The listing builds one solid part. Answer for the finished solid, in the listing's coordinates (mm). A direction names the side the tool comes from. Coordinates: 2 decimals unless noted, no trailing zeros. Write each loop counter-clockwise with the first axis right and the second up, starting at its lowest first coordinate (ties: lowest second). Pieces come first, ordered by that corner, then holes. Notation, with made-up numbers: M 19.25,62.25 L 71.25,62.25 A16 ccw 71.25,83.25 Z; hole C 23.25,-4 d6. An arc over 180 degrees is marked long. Write item = value, one per line. Start each with the question number.
```python
from build123d import *

# Parameters (mm, degrees)
EXTRUDE_1_DEPTH     = 3
SKETCH_3_W          = 60
SKETCH_3_H          = 31.5
EXTRUDE_2_DEPTH     = 2
SKETCH_4_R          = 0.5
CUT_EXTRUDE_1_DEPTH = 10
SKETCH_5_R          = 1.5
CUT_EXTRUDE_2_DEPTH = 10
SKETCH_6_W          = 5
SKETCH_6_H          = 31.5
EXTRUDE_3_DEPTH     = 48.15
EXTRUDE_START       = 5
SKETCH_7_R          = 1.6
EXTRUDE_4_DEPTH     = 5
CUT_EXTRUDE_3_DEPTH = 2
FILLET_1_R          = 2
FILLET_2_R          = 2
CUT_EXTRUDE_5_DEPTH = 1.6
SKETCH_11_R         = 0.5
SKETCH_11_R_2       = 1.5
EXTRUDE_5_DEPTH     = 3
SKETCH_12_W         = 31.5
SKETCH_12_H         = 1.6
EXTRUDE_6_DEPTH     = 9
FILLET_4_R          = 1.6
EXTRUDE_START_2     = 1.6
SKETCH_13_R         = 10
SKETCH_13_R_2       = 1.75
SKETCH_13_R_3       = 0.5
EXTRUDE_7_DEPTH     = 1.6
SKETCH_14_R         = 1.6
CUT_EXTRUDE_6_DEPTH = 67.6


with BuildPart() as part:
    # 草图1 → 凸台-拉伸1 (new body)
    with BuildSketch(Plane(origin=(0, 0, 0), x_dir=(1, 0, 0), z_dir=(0, 1, 0))):
        with BuildLine():
            Line((0, -15.75), (90, -15.75))
            Line((90, -15.75), (90, 15.75))
            Line((90, 15.75), (0, 15.75))
            ThreePointArc((0, 15.75), (-15.75, 0), (0, -15.75))
        make_face()
    extrude(amount=EXTRUDE_1_DEPTH)

    # 草图3 → 凸台-拉伸2 (add)
    with BuildSketch(Plane.XZ):
        with Locations((60, 0)):
            Rectangle(SKETCH_3_W, SKETCH_3_H)
    extrude(amount=EXTRUDE_2_DEPTH)

    # 草图4 → 切除-拉伸1 (cut)
    with BuildSketch(Plane.XZ):
        with Locations(Location((0, 7, 0), (0, 0, 270))):
            Circle(SKETCH_4_R)
        with Locations(Location((7, 0, 0), (0, 0, 270))):
            Circle(SKETCH_4_R)
        with Locations(Location((0, -7, 0), (0, 0, 270))):
            Circle(SKETCH_4_R)
        with Locations(Location((-7, 0, 0), (0, 0, 270))):
            Circle(SKETCH_4_R)
    extrude(amount=-CUT_EXTRUDE_1_DEPTH, mode=Mode.SUBTRACT)

    # 草图5 → 切除-拉伸2 (cut)
    with BuildSketch(Plane(origin=(0, 3, 0), x_dir=(1, 0, 0), z_dir=(0, 1, 0))):
        with Locations(Location((0, 0, 0), (0, 0, 270))):
            Circle(SKETCH_5_R)
    extrude(amount=-CUT_EXTRUDE_2_DEPTH, mode=Mode.SUBTRACT)

    # 草图6 → 凸台-拉伸3 (add)
    with BuildSketch(Plane.XZ.offset(2)):
        with Locations((87.5, 0)):
            Rectangle(SKETCH_6_W, SKETCH_6_H)
    extrude(amount=EXTRUDE_3_DEPTH)

    # 草图7 → 凸台-拉伸4 (add)
    with BuildSketch(Plane.XZ.offset(50.15).offset(EXTRUDE_START)):
        with BuildLine():
            Line((90, 15.75), (0, 15.75))
            ThreePointArc((0, 15.75), (-15.75, 0), (0, -15.75))
            Line((0, -15.75), (90, -15.75))
            Line((90, -15.75), (90, 15.75))
        make_face()
        with Locations(Location((8.03393099, 0, 0), (0, 0, 270))):
            Circle(SKETCH_7_R, mode=Mode.SUBTRACT)
        with Locations(Location((0, 8, 0), (0, 0, 270))):
            Circle(SKETCH_7_R, mode=Mode.SUBTRACT)
        with Locations(Location((0.03393099, -7.999928043, 0), (0, 0, 270))):
            Circle(SKETCH_7_R, mode=Mode.SUBTRACT)
        with Locations(Location((-8, 0, 0), (0, 0, 270))):
            Circle(SKETCH_7_R, mode=Mode.SUBTRACT)
    extrude(amount=-EXTRUDE_4_DEPTH)

    # 草图8 → 切除-拉伸3 (cut)
    with BuildSketch(Plane(origin=(0, -50.15, 0), x_dir=(1, 0, 0), z_dir=(0, 1, 0))):
        Polygon((0, 15.75), (30, 15.75), (30, -15.75), (0, -15.75), (-20, -15.75), (-20, 15.75), align=None)
    extrude(amount=-CUT_EXTRUDE_3_DEPTH, mode=Mode.SUBTRACT)

    # 圆角1
    fillet_1_edges = [part.edges().sort_by_distance(p)[0] for p in [
        (85, -2, 0),
    ]]
    fillet(fillet_1_edges, radius=FILLET_1_R)

    # 圆角2
    fillet_2_edges = [part.edges().sort_by_distance(p)[0] for p in [
        (85, -50.15, 0),
    ]]
    fillet(fillet_2_edges, radius=FILLET_2_R)

    # 草图10 → 切除-拉伸5 (cut)
    with BuildSketch(Plane.XZ):
        with BuildLine():
            Line((30, -15.75), (30, 15.75))
            Line((30, 15.75), (0, 15.75))
            ThreePointArc((0, 15.75), (-15.75, 0), (0, -15.75))
            Line((0, -15.75), (30, -15.75))
        make_face()
    extrude(amount=-CUT_EXTRUDE_5_DEPTH, mode=Mode.SUBTRACT)

    # 草图11 → 凸台-拉伸5 (add)
    with BuildSketch(Plane.XZ.offset(-1.6)):
        with BuildLine():
            Line((0, -15.75), (30, -15.75))
            Line((30, -15.75), (30, 15.75))
            Line((30, 15.75), (0, 15.75))
            ThreePointArc((0, 15.75), (-15.75, 0), (0, -15.75))
        make_face()
        with Locations(Location((0, -7, 0), (0, 0, 270))):
            Circle(SKETCH_11_R, mode=Mode.SUBTRACT)
        with Locations(Location((-7, 0, 0), (0, 0, 270))):
            Circle(SKETCH_11_R, mode=Mode.SUBTRACT)
        with Locations(Location((0, 0, 0), (0, 0, 270))):
            Circle(SKETCH_11_R_2, mode=Mode.SUBTRACT)
        with Locations(Location((0, 7, 0), (0, 0, 270))):
            Circle(SKETCH_11_R, mode=Mode.SUBTRACT)
        with Locations(Location((7, 0, 0), (0, 0, 270))):
            Circle(SKETCH_11_R, mode=Mode.SUBTRACT)
    extrude(amount=-EXTRUDE_5_DEPTH)

    # 草图12 → 凸台-拉伸6 (add)
    with BuildSketch(Plane(origin=(30, 0, 0), x_dir=(0, 0, -1), z_dir=(1, 0, 0))):
        with Locations((0, 3.8)):
            Rectangle(SKETCH_12_W, SKETCH_12_H)
    extrude(amount=EXTRUDE_6_DEPTH)

    # 圆角4
    fillet_4_edges = [part.edges().sort_by_distance(p)[0] for p in [
        (39, 3, 0),
    ]]
    fillet(fillet_4_edges, radius=FILLET_4_R - 0.0001)  # a hair under: the kernel refuses the full size

    # 草图13 → 凸台-拉伸7 (add)
    with BuildSketch(Plane.XZ.offset(-1.6).offset(EXTRUDE_START_2)):
        with Locations(Location((0, 0, 0), (0, 0, 270))):
            Circle(SKETCH_13_R)
        with Locations(Location((0, 0, 0), (0, 0, 270))):
            Circle(SKETCH_13_R_2, mode=Mode.SUBTRACT)
        with Locations(Location((7, 0, 0), (0, 0, 270))):
            Circle(SKETCH_13_R_3, mode=Mode.SUBTRACT)
        with Locations(Location((0, -7, 0), (0, 0, 270))):
            Circle(SKETCH_13_R_3, mode=Mode.SUBTRACT)
        with Locations(Location((-7, 0, 0), (0, 0, 270))):
            Circle(SKETCH_13_R_3, mode=Mode.SUBTRACT)
        with Locations(Location((0, 7, 0), (0, 0, 270))):
            Circle(SKETCH_13_R_3, mode=Mode.SUBTRACT)
    extrude(amount=-EXTRUDE_7_DEPTH)

    # 草图14 → 切除-拉伸6 (cut)
    with BuildSketch(Plane.XZ.offset(55.15)):
        with Locations(Location((68.4, 0, 0), (0, 0, 270))):
            Circle(SKETCH_14_R)
        with Locations(Location((78.4, 0, 0), (0, 0, 270))):
            Circle(SKETCH_14_R)
    extrude(amount=-CUT_EXTRUDE_6_DEPTH, mode=Mode.SUBTRACT)


solid = part.part
```
1. For faces 4 (the face through (-9.56, -53.67, 0.35)), 5 (the face through (30, -51, 0)), 6 (the face through (30, 0, 0)), 7 (the face through (-1.71, 0.79, 0.38)), determine the directions among +Z, -Z, +X, -X, +Y, -Y from which every point of the face is accessible in a straight line to the end or side of a thin tool.
2. Straight lines are drawn through the part: L1, parallel to Y at x = -7, z = 13; L2, parallel to X at y = -53.5, z = 0; L3, parallel to Z at x = 68.4, y = -54. For each, find the intervals that lie inside material, in ascending order. Write a range as [from, to].
3. The part is cut by section D-D, the plane y = -13. Write down the section's boundary in (x, z), and give its area (4 significant figures).
4. The part is cut by section B-B, the plane x = 78.4. Write down the section's boundary in (y, z), and give its area (3 significant figures).
5. The part is cut by section C-C, the plane x = 54.5. Write down the section's boundary in (y, z).
6. The part is cut by section A-A, the plane x = 25.5. Write down the section's boundary in (y, z), and give its area (3 significant figures).
7. For a pull along Z with two mould halves and no side action, classify faces 1 (the face through (84.43, -2.6, 0.22)), 2 (the face through (-15.746, -53.671, 0.346)), 3 (the face through (76.84, -52.68, 0.35)) as pulls with the +Z half, pulls with the -Z half, needs draft (parallel to the pull), parting line crosses it, or undercut.
8. Each of these flat-tipped pins is pushed along its axis until it touches: pin 1 (3.5 mm diameter, centred on x = 68.4, z = 0, fed in from -Y); pin 2 (2.5 mm diameter, centred on x = 0, z = 0, fed in from +Y); pin 3 (3.5 mm diameter, centred on x = 68.4, z = 0, fed in from +Y); pin 4 (3 mm diameter, centred on x = 0, z = 8, fed in from -Y). Where does it stop, or does it pass through?
Solution:
q1.face_4 = -Y
q1.face_5 = +Z, -Z, -X
q1.face_6 = +Z, -Z
q1.face_7 = none
q2.L1 = [-55.15, -52.15], [1.6, 4.6]
q2.L2 = [-15.75, -9.6], [-6.4, 6.43], [9.63, 66.8], [70, 76.8], [80, 90]
q2.L3 = [-15.75, -1.6], [1.6, 15.75]
q3.outline = M 85,-15.75 L 90,-15.75 L 90,15.75 L 85,15.75 Z
q3.area = 157.5 mm^2
q4.outline = M -55.15,-15.75 L -50.15,-15.75 L -50.15,-1.6 L -55.15,-1.6 Z; M -55.15,1.6 L -50.15,1.6 L -50.15,15.75 L -55.15,15.75 Z; M -2,-15.75 L 3,-15.75 L 3,-1.6 L -2,-1.6 Z; M -2,1.6 L 3,1.6 L 3,15.75 L -2,15.75 Z
q4.area = 283 mm^2
q5.outline = M -55.15,-15.75 L -50.15,-15.75 L -50.15,15.75 L -55.15,15.75 Z; M -2,-15.75 L 3,-15.75 L 3,15.75 L -2,15.75 Z
q6.outline = M -55.15,-15.75 L -52.15,-15.75 L -52.15,15.75 L -55.15,15.75 Z; M 1.6,-15.75 L 4.6,-15.75 L 4.6,15.75 L 1.6,15.75 Z
q6.area = 189 mm^2
q7.face_1 = needs draft
q7.face_2 = parting line crosses it
q7.face_3 = undercut
q8.pin_1 = -55.15
q8.pin_2 = -52.15
q8.pin_3 = 3
q8.pin_4 = 0
